```python
from build123d import *

# Parameters (mm, degrees)
PAD_DEPTH    = 3
FILLET_R     = 100
FILLET001_R  = 3
SKETCH001_R  = 2.25
POCKET_DEPTH = 5


with BuildPart() as part:
    # Sketch → Pad (new body)
    with BuildSketch(Plane.XY):
        with BuildLine():
            Line((-5, 12.5), (5, 12.5))
            Line((5, 12.5), (5, -12.5))
            Line((0.877121, -35.882006), (5, -12.5))
            ThreePointArc((-0.877121, -35.882006), (0, -36.617999), (0.877121, -35.882006))
            Line((-5, -12.5), (-0.877121, -35.882006))
            Line((-5, -12.5), (-5, 12.5))
        make_face()
    extrude(amount=PAD_DEPTH)

    # Fillet
    fillet_edges = [part.edges().sort_by_distance(p)[0] for p in [
        (5, -12.5, 1.5),
        (-5, -12.5, 1.5),
    ]]
    fillet(fillet_edges, radius=FILLET_R)

    # Fillet001
    fillet001_edges = [part.edges().sort_by_distance(p)[0] for p in [
        (5, 12.5, 1.5),
        (-5, 12.5, 1.5),
    ]]
    fillet(fillet001_edges, radius=FILLET001_R)

    # Sketch001 (on Face5 of Fillet001) → Pocket (cut)
    with BuildSketch(Plane.XY.offset(3)):
        with Locations((0, 8.5)):
            Circle(SKETCH001_R)
    extrude(amount=-POCKET_DEPTH, mode=Mode.SUBTRACT)


solid = part.part
```
Read the model definition and answer for the solid it produces. Units are mm, in the model's axes. Coordinates: 2 decimals unless noted, no trailing zeros. Order: outer loops, then holes, each group sorted by start corner. A loop starts at its lowest first (then second) coordinate and runs counter-clockwise, first axis right, second up. Notation, with made-up numbers: (45, 36.25) - (75, 36.25) arc R23 ccw to (75, 64.25) - close; hole circle Ø10 at (17.25, -38.75). An arc over 180 degrees is marked (long way). Answer as a JSON object with one key per item and string values. Group by question number.
Item 1: Section B-B (y = 8.5) is taken. Give the vertices of the cut face in (x, z).
Item 2: Section D-D (y = -18) is taken. Give the vertices of the cut face in (x, z), plus the area to 3 significant figures.
Item 3: Section C-C (z = 1.1) is taken. Give the vertices of the cut face in (x, y).
Item 4: Section A-A (x = 0) is taken. Give the vertices of the cut face in (y, z), plus the area to 3 significant figures.
Item 5: The mould has two halves that part along X. Classify faces 1 (the face through (-5, 3, 1)), 2 (the face through (-0.29, 10.73, 1.52)), 3 (the face through (0, -6, 3)): +X half, -X half, draft (parallel to the pull), parting line (faces both ways), or undercut.
Item 6: Consider probe 1 along Y at (x, z) = (0, 1.1); probe 2 along Y at (x, z) = (-0.5, 2.7); probe 3 along X at (y, z) = (-17, 0.35). Determine where each line is inside the solid, lowest interval first. Write a range as from..to.
Results are:
{
 "1": {"outline": "(-5, 0) - (-2.25, 0) - (-2.25, 3) - (-5, 3) - close; (2.25, 0) - (5, 0) - (5, 3) - (2.25, 3) - close"},
 "2": {"outline": "(-3.98, 0) - (3.98, 0) - (3.98, 3) - (-3.98, 3) - close", "area": "23.9 mm^2"},
 "3": {"outline": "(-5, -3.75) arc R100 ccw to (-3.48, -21.12) - (-0.88, -35.88) arc R0.89 ccw to (0.88, -35.88) - (3.48, -21.12) arc R100 ccw to (5, -3.75) - (5, 9.5) arc R3 ccw to (2, 12.5) - (-2, 12.5) arc R3 ccw to (-5, 9.5) - close; hole circle Ø4.5 at (0, 8.5)"},
 "4": {"outline": "(-36.62, 0) - (6.25, 0) - (6.25, 3) - (-36.62, 3) - close; (10.75, 0) - (12.5, 0) - (12.5, 3) - (10.75, 3) - close", "area": "134 mm^2"},
 "5": {"face 1": "-X half", "face 2": "undercut", "face 3": "draft"},
 "6": {"probe 1": "y = -36.62..6.25, 10.75..12.5", "probe 2": "y = -36.46..6.31, 10.69..12.5", "probe 3": "x = -4.12..4.12"}
}
